```python
from build123d import *

# Parameters (mm, degrees)
F2_R = 6.34999


# Not quite as in the source:
# - a fillet or chamfer is up to 0.001 mm smaller than in the source, because OpenCascade refuses the exact size


with BuildPart() as f1:
    # F0 (on Front) → F1 (revolve)
    with BuildSketch(Plane.XZ):
        Polygon((3.9624, -2.38125), (0, -2.38125), (0, -19.85645), (113.5126, -19.85645), (113.5126, -13.50645), (3.9624, -13.50645), align=None)
    revolve(axis=Axis((1.9812, 0, -2.38125), (-1, 0, 0)))

    # F2 (radius 6.35 in the source; OpenCascade refuses exactly that, so slightly less here)
    f2_edges = [f1.edges().sort_by_distance(p)[0] for p in [
        (0, 0, 15.09395),
        (113.5126, 0, 15.09395),
        (56.7563, 0, -19.85645),
    ]]
    fillet(f2_edges, radius=F2_R)


solid = f1.part
```
Geometry check sheet. Reference: the model listing, model coordinates, mm. Coordinates: 2 decimals unless noted, no trailing zeros. Write each loop counter-clockwise with the first axis right and the second up, starting at its lowest first coordinate (ties: lowest second). Pieces come first, ordered by that corner, then holes. Notation, with made-up numbers: M -34,30.25 L -12,30.25 A22 cw -12,42.25 Z; hole C 46.25,24.5 d6. An arc over 180 degrees is marked long. Answer as a JSON object with one key per item and string values.
1. Section check B-B, the plane x = 15. Enter the section's corners in (y, z), plus the area to 3 significant figures.
Answers below:
{"outline": "C 0,-2.38 d34.95; hole C 0,-2.38 d22.25", "area": "571 mm²"}
2. Go/stop test with flat-tipped pins: pin 1 Ø10 at (y, z) = (1.5, 2) entering from -X; pin 2 Ø3 at (x, z) = (59, -9) entering from +Y; pin 3 Ø20 at (y, z) = (0, -2.38) entering from +X; pin 4 Ø2 at (x, y) = (14, -8) entering from +Z. Record where each tip stops, or that it passes through.
Answers below:
{"pin 1": "stops at x = 0", "pin 2": "stops at y = 16.71", "pin 3": "stops at x = 3.96", "pin 4": "stops at z = 13.63"}
3. Draft check along Y on faces 1 (the cylindrical face through (57.46, -5.25, -19.05)), 2 (the flat face through (0, 0, -3)), 3 (the flat face through (3.962, 0, -2)). Enter one of: released by +Y, released by -Y, zero draft, split by the parting line, or undercut.
Answers below:
{"face 1": "split by the parting line", "face 2": "zero draft", "face 3": "undercut"}
4. Scan lines: L1, parallel to Y at x = 44, z = -3; L2, parallel to Z at x = 52, y = 0; L3, parallel to Z at x = 87, y = 4. Record each from-to range of solid material in increasing order.
Answers below:
{"L1": "y = -17.46 to -11.11, 11.11 to 17.46", "L2": "z = -19.86 to -13.51, 8.74 to 15.09", "L3": "z = -19.39 to -12.76, 8 to 14.63"}
